Here's how the part is built. I have some questions about the finished solid (model axes, mm). A direction names the side the tool comes from. Give positions to 0.01 mm unless a question says otherwise; leave off trailing zeros. Loops run counter-clockwise (first coordinate to the right, second up) from the corner with the lowest first, then second, coordinate; pieces in that order, holes last.
Q1. Will these pins go through, and if not, where does the flat tip stop? P1, Ø5.5, axis at x = 34.925, z = 6.35, coming from the +Y side; P2, Ø6, axis at y = 35, z = 7, coming from the +X side (3 decimals); P3, Ø2, axis at x = 27.5, z = 11, coming from the +Y side; P4, Ø3.5, axis at x = 32, z = 5.5, coming from the -Y side.
Q2. For faces 5 (the face through (41.275, 7, 6)), 6 (the face through (12, 28, 12.7)), 7 (the face through (30, -0.508, 6)), 8 (the face through (32, -12.7, 4)), 9 (the face through (32, 12.7, 4)), which set-ups out of +Z, -Z, +X, -X, +Y, -Y let a thin tool reach every point of the face, with its end or its side?
Q3. If we section it at A-A (x = -7.62): Please give me the cut outline in (y, z).
Q4. If we section it at D-D (x = -19.05): Please give me the cut outline in (y, z), plus the area to 3 significant figures.
Q5. We'd pull the mould along X, two halves only. Please class faces 1 (the face through (18, 11, 0)), 2 (the face through (-41.275, -1, 6)), 3 (the face through (-18.394, 39.924, 4.344)), 4 (the face through (26.94, 13.655, 6.261)): +X half, -X half, draft (parallel to the pull), parting line (faces both ways), or undercut.
Q6. If we section it at C-C (z = 6.35): Please give me the cut outline in (x, y) (3 decimals).
Q7. I need wall thicknesses on line 1 (Y direction, x = -19.05, z = 3); line 2 (X direction, y = 7, z = 3.25) (1 decimal); line 3 (Y direction, x = -7.62, z = 4). Which ranges of each line are inside material? Lowest first, please.
Q8. If we section it at B-B (y = -6): Please give me the cut outline in (x, z) (3 decimals).
from build123d import *

# Parameters (mm, degrees)
SKETCH1_W                                           = 82.55
SKETCH1_H                                           = 88.9
EXTRUDE1_DEPTH                                      = 12.7
SKETCH2_R                                           = 27.1272
EXTRUDE2_DEPTH                                      = 13.7
SKETCH3_W                                           = 28.468633454
SKETCH3_H                                           = 1.016
EXTRUDE3_DEPTH                                      = 13.7
F_1_4_CLEARANCE_HOLE1_D                             = 6.7564
CSK_FOR_3_8_FLAT_HEAD_MACHINE_SCREW_100_D           = 10.0838
CSK_FOR_3_8_FLAT_HEAD_MACHINE_SCREW_100_CSINK_D     = 19.3548
CSK_FOR_3_8_FLAT_HEAD_MACHINE_SCREW_100_CSINK_ANGLE = 100
SKETCH10_W                                          = 15.24
SKETCH10_H                                          = 31.75
EXTRUDE4_DEPTH                                      = 13.7000001
FILLET1_R                                           = 3.175


with BuildPart() as part:
    # Sketch1 → Extrude1 (new body)
    with BuildSketch(Plane.XY):
        Rectangle(SKETCH1_W, SKETCH1_H)
    extrude(amount=EXTRUDE1_DEPTH)

    # Sketch2 → Extrude2 (cut, through all)
    with BuildSketch(Plane.XY.offset(12.7)):
        with Locations((-7.62, 0)):
            Circle(SKETCH2_R)
    extrude(amount=-EXTRUDE2_DEPTH, mode=Mode.SUBTRACT)

    # Sketch3 → Extrude3 (cut, through all)
    with BuildSketch(Plane.XY.offset(12.7)):
        with Locations((30.3911, 0)):
            Rectangle(SKETCH3_W, SKETCH3_H)
    extrude(amount=-EXTRUDE3_DEPTH, mode=Mode.SUBTRACT)

    # 1/4 Clearance Hole1 (through all)
    with Locations(Plane(origin=(34.925, 44.45, 6.35), x_dir=(0, 0, 1), z_dir=(0, 1, 0))):
        with Locations((0, 0)):
            Hole(F_1_4_CLEARANCE_HOLE1_D / 2)

    # CSK for 3/8 Flat Head Machine Screw (100)1 (through all)
    with Locations(Plane(origin=(-19.05, 34.925, 12.7), x_dir=(1, 0, 0), z_dir=(0, 0, 1))):
        with Locations((0, 0)):
            csk_for_3_8_flat_head_machine_screw_100 = CounterSinkHole(CSK_FOR_3_8_FLAT_HEAD_MACHINE_SCREW_100_D / 2, CSK_FOR_3_8_FLAT_HEAD_MACHINE_SCREW_100_CSINK_D / 2, counter_sink_angle=CSK_FOR_3_8_FLAT_HEAD_MACHINE_SCREW_100_CSINK_ANGLE)

    # Mirror1: CSK for 3/8 Flat Head Machine Screw (100)1 across plane
    add(csk_for_3_8_flat_head_machine_screw_100.mirror(Plane.ZX), mode=Mode.SUBTRACT)

    # Sketch10 → Extrude4 (cut, through all)
    with BuildSketch(Plane.XY.offset(12.7)):
        with Locations((33.655, 28.575)):
            Rectangle(SKETCH10_W, SKETCH10_H)
    extrude4 = extrude(amount=-EXTRUDE4_DEPTH, mode=Mode.SUBTRACT)

    # Mirror2: Extrude4 across plane
    add(extrude4.mirror(Plane.ZX), mode=Mode.SUBTRACT)

    # Fillet1
    fillet1_edges = [part.edges().sort_by_distance(p)[0] for p in [
        (26.035, 12.7, 6.35),
        (26.035, -12.7, 6.35),
    ]]
    fillet(fillet1_edges, radius=FILLET1_R)


solid = part.part
Check sheet entries:
1. P1: passes through
1. P2: stops at x = 26.035
1. P3: stops at y = 14.22
1. P4: stops at y = -12.7
2. face 5: +Z, -Z, +X, +Y, -Y
2. face 6: +Z, +X, -X, +Y, -Y
2. face 7: +Z, -Z, +X
2. face 8: +Z, -Z, +X, -Y
2. face 9: +Z, -Z, +X, +Y
3. outline: (-44.45, 0) - (-27.13, 0) - (-27.13, 12.7) - (-44.45, 12.7) - close; (27.13, 0) - (44.45, 0) - (44.45, 12.7) - (27.13, 12.7) - close
4. outline: (-44.45, 0) - (-39.97, 0) - (-39.97, 8.81) - (-44.45, 12.57) - close; (-29.88, 0) - (-24.6, 0) - (-24.6, 12.7) - (-25.25, 12.7) - (-29.88, 8.81) - close; (24.6, 0) - (29.88, 0) - (29.88, 8.81) - (25.25, 12.7) - (24.6, 12.7) - close; (39.97, 0) - (44.45, 0) - (44.45, 12.57) - (39.97, 8.81) - close
4. area: 212 mm2
5. face 1: draft
5. face 2: -X half
5. face 3: undercut
5. face 4: +X half
6. outline: (-41.275, -44.45) - (26.035, -44.45) - (26.035, -15.875) arc R3.175 cw to (29.21, -12.7) - (31.547, -12.7) - (31.547, -0.508) - (19.502, -0.508) arc R27.127 cw (long way) to (19.502, 0.508) - (31.547, 0.508) - (31.547, 12.7) - (29.21, 12.7) arc R3.175 cw to (26.035, 15.875) - (26.035, 44.45) - (-41.275, 44.45) - close; (38.303, -12.7) - (41.275, -12.7) - (41.275, -0.508) - (38.303, -0.508) - close; (38.303, 0.508) - (41.275, 0.508) - (41.275, 12.7) - (38.303, 12.7) - close; hole circle Ø10.084 at (-19.05, -34.925); hole circle Ø10.084 at (-19.05, 34.925)
7. line 1: y = -44.45 to -39.97, -29.88 to -24.6, 24.6 to 29.88, 39.97 to 44.45
7. line 2: x = -41.3 to -33.8, 18.6 to 33.6, 36.3 to 41.3
7. line 3: y = -44.45 to -27.13, 27.13 to 44.45
8. outline: (-41.275, 0) - (-34.075, 0) - (-34.075, 12.7) - (-41.275, 12.7) - close; (18.835, 0) - (41.275, 0) - (41.275, 12.7) - (18.835, 12.7) - close; hole circle Ø6.756 at (34.925, 6.35)
